The model under review builds one solid part; all positions refer to its coordinate system, in mm. Round coordinates to 2 decimals unless told otherwise and drop trailing zeros. Write each loop counter-clockwise with the first axis right and the second up, starting at its lowest first coordinate (ties: lowest second). Pieces come first, ordered by that corner, then holes. Notation, with made-up numbers: (50, -31) - (102, -31) arc R23 cw to (102, -11) - close; hole circle Ø7 at (-2, -14). An arc over 180 degrees is marked (long way). Write each question's results on one line, items separated by ' | '.
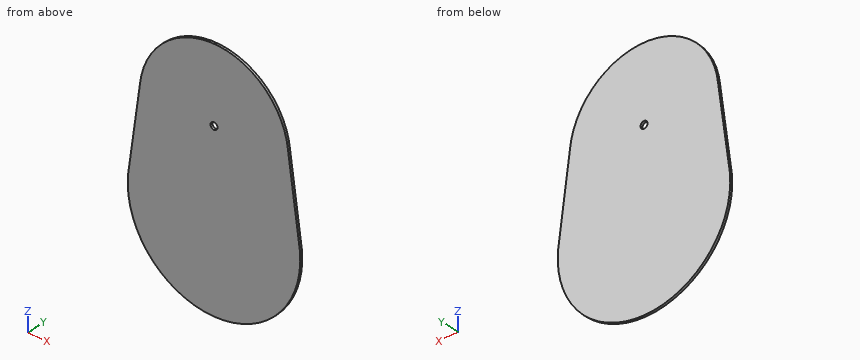
```python
from build123d import *

# Parameters (mm, degrees)
F1_DEPTH = 3
F2_R     = 4.5
F3_DEPTH = 3.001


with BuildPart() as f1:
    # F0 (on Front) → F1 (new body)
    with BuildSketch(Plane.XZ):
        with BuildLine():
            Line((108.20451, -90.206463), (94.563775, 9.093536))
            ThreePointArc((94.563775, 9.093536), (0, 95), (-94.563775, 9.093536))
            Line((-94.563775, 9.093536), (-108.20451, -90.206463))
            Line((-108.20451, -90.206463), (-109.533774, -99.883063))
            ThreePointArc((-109.533774, -99.883063), (0, -220), (109.533774, -99.883063))
            Line((109.533774, -99.883063), (108.20451, -90.206463))
        make_face()
    extrude(amount=F1_DEPTH)

    # F2 (on face) → F3 (cut, through all)
    with BuildSketch(Plane.XZ.offset(3)):
        Circle(F2_R)
    extrude(amount=-F3_DEPTH, mode=Mode.SUBTRACT)


solid = f1.part
```
Q1. Insertion check: P1, Ø7, axis at x = 0, z = 0, coming from the -Y side; P2, Ø1, axis at y = -2, z = -0.5, coming from the -X side. Each pin has a flat end and moves straight along its axis. Give the tip position at first contact, or say it passes through.
Evaluation:
P1: passes through | P2: stops at x = -95.95
Q2. We need section C-C (z = 0). State the section outline as (x, y) points, plus the area to 3 significant figures.
Evaluation:
outline: (-95.81, -3) - (-4.5, -3) - (-4.5, 0) - (-95.81, 0) - close; (4.5, -3) - (95.81, -3) - (95.81, 0) - (4.5, 0) - close | area: 548 mm^2
Q3. We need section B-B (y = -1.5). State the section outline as (x, z) points.
Evaluation:
outline: (-109.53, -99.88) arc R110 ccw (long way) to (109.53, -99.88) - (94.56, 9.09) arc R95 ccw to (-94.56, 9.09) - close; hole circle Ø9 at (0, 0)
Q4. We need section A-A (x = 0). State the section outline as (y, z) points.
Evaluation:
outline: (-3, -220) - (0, -220) - (0, -4.5) - (-3, -4.5) - close; (-3, 4.5) - (0, 4.5) - (0, 95) - (-3, 95) - close
Q5. For probe 1 along Z at (x, y) = (0, -2); probe 2 along Z at (x, y) = (-1, -0.85); probe 3 along X at (y, z) = (-0.3, -108.5), list the stretches that pass through material, from the lowest coordinate up.
Evaluation:
probe 1: z = -220 to -4.5, 4.5 to 95 | probe 2: z = -220 to -4.39, 4.39 to 94.99 | probe 3: x = -109.99 to 109.99
Q6. We need section D-D (x = 91). State the section outline as (y, z) points.
Evaluation:
outline: (-3, -171.8) - (0, -171.8) - (0, 27.28) - (-3, 27.28) - close
